```python
from build123d import *

# Parameters (mm, degrees)
BOSS_EXTRUDE1_DEPTH           = 1.8
EXTRUDE_THIN1_START           = 1.8
EXTRUDE_THIN1_DEPTH           = 3
SKETCH7_R                     = 1.55
SKETCH7_R_2                   = 0.01
EXTRUDE_THIN2_DEPTH           = 3.2
EXTRUDE_THIN2_DRAFT           = 5
EXTRUDE_THIN2_PROFILE_2_DEPTH = 3.2
EXTRUDE_THIN2_PROFILE_2_DRAFT = 5
EXTRUDE_THIN2_PROFILE_3_DEPTH = 3.2
EXTRUDE_THIN2_PROFILE_3_DRAFT = 5
EXTRUDE_THIN2_PROFILE_4_DEPTH = 3.2
EXTRUDE_THIN2_PROFILE_4_DRAFT = 5


with BuildPart() as part:
    # Sketch1 → Boss-Extrude1 (new body)
    with BuildSketch(Plane(origin=(0, 0, 0), x_dir=(0, 1, 0), z_dir=(0, 0, 1))):
        Polygon((40.609900374, 53.452613812), (-31.190099626, 53.452613812), (-31.190099626, -5.547386188), (40.609900374, -5.547386188), (40.609900374, -0.297386188), (43.209900374, 2.202613812), (43.109900374, 34.902613812), (40.609900374, 37.502613812), align=None)
    extrude(amount=BOSS_EXTRUDE1_DEPTH)

    # Sketch5 → Extrude-Thin1 (add)
    with BuildSketch(Plane(origin=(0, 0, 0), x_dir=(0, 1, 0), z_dir=(0, 0, 1)).offset(EXTRUDE_THIN1_START)):
        Polygon((-29.390099626, 51.652613812), (-29.390099626, -3.747386188), (38.809900374, -3.747386188), (38.809900374, -0.88342499), (41.360418353, 1.616884702), (41.360418353, 35.141633158), (38.809900374, 37.64194285), (38.809900374, 51.652613812), align=None)
        Polygon((-28.590099626, 50.852613812), (-28.590099626, -2.947386188), (38.009900374, -2.947386188), (38.009900374, -0.547386188), (40.560418353, 1.952923505), (40.560418353, 34.805594355), (38.009900374, 37.305904047), (38.009900374, 50.852613812), align=None, mode=Mode.SUBTRACT)
    extrude(amount=EXTRUDE_THIN1_DEPTH)


with BuildPart() as extrude_thin2_tool:
    # Sketch7 → Extrude-Thin2 (with draft: the straight prism first)
    with BuildSketch(Plane.XY.offset(1.8)):
        with Locations((-4.802613812, 37.960418353)):
            Circle(SKETCH7_R)
        with Locations((-4.802613812, 37.960418353)):
            Circle(SKETCH7_R_2, mode=Mode.SUBTRACT)
    extrude(amount=EXTRUDE_THIN2_DEPTH)
    # Extrude-Thin2: the draft: its side faces are tilted about the plane it starts from
    extrude_thin2_sides = [extrude_thin2_tool.faces().sort_by_distance(p)[0] for p in [
        (-6.352613812, 37.960418353, 3.4),
        (-4.812613812, 37.960418353, 3.4),
    ]]
    draft(extrude_thin2_sides, Plane.XY.offset(1.8), EXTRUDE_THIN2_DRAFT)


with BuildPart() as part_1:
    add(part.part)

    # Extrude-Thin2: add extrude_thin2_tool
    add(extrude_thin2_tool.part)


with BuildPart() as extrude_thin2_profile_2_tool:
    # Sketch7 → Extrude-Thin2 profile 2 (with draft: the straight prism first)
    with BuildSketch(Plane.XY.offset(1.8)):
        with Locations((-32.702613812, 37.960418353)):
            Circle(SKETCH7_R)
        with Locations((-32.702613812, 37.960418353)):
            Circle(SKETCH7_R_2, mode=Mode.SUBTRACT)
    extrude(amount=EXTRUDE_THIN2_PROFILE_2_DEPTH)
    # Extrude-Thin2 profile 2: the draft: its side faces are tilted about the plane it starts from
    extrude_thin2_profile_2_sides = [extrude_thin2_profile_2_tool.faces().sort_by_distance(p)[0] for p in [
        (-34.252613812, 37.960418353, 3.4),
        (-32.712613812, 37.960418353, 3.4),
    ]]
    draft(extrude_thin2_profile_2_sides, Plane.XY.offset(1.8), EXTRUDE_THIN2_PROFILE_2_DRAFT)


with BuildPart() as part_2:
    add(part_1.part)

    # Extrude-Thin2 profile 2: add extrude_thin2_profile_2_tool
    add(extrude_thin2_profile_2_tool.part)


with BuildPart() as extrude_thin2_profile_3_tool:
    # Sketch7 → Extrude-Thin2 profile 3 (with draft: the straight prism first)
    with BuildSketch(Plane.XY.offset(1.8)):
        with Locations((0.297386188, -14.140099626)):
            Circle(SKETCH7_R)
        with Locations((0.297386188, -14.140099626)):
            Circle(SKETCH7_R_2, mode=Mode.SUBTRACT)
    extrude(amount=EXTRUDE_THIN2_PROFILE_3_DEPTH)
    # Extrude-Thin2 profile 3: the draft: its side faces are tilted about the plane it starts from
    extrude_thin2_profile_3_sides = [extrude_thin2_profile_3_tool.faces().sort_by_distance(p)[0] for p in [
        (-1.252613812, -14.140099626, 3.4),
        (0.287386188, -14.140099626, 3.4),
    ]]
    draft(extrude_thin2_profile_3_sides, Plane.XY.offset(1.8), EXTRUDE_THIN2_PROFILE_3_DRAFT)


with BuildPart() as part_3:
    add(part_2.part)

    # Extrude-Thin2 profile 3: add extrude_thin2_profile_3_tool
    add(extrude_thin2_profile_3_tool.part)


with BuildPart() as extrude_thin2_profile_4_tool:
    # Sketch7 → Extrude-Thin2 profile 4 (with draft: the straight prism first)
    with BuildSketch(Plane.XY.offset(1.8)):
        with Locations((-48.102613812, -13.040099626)):
            Circle(SKETCH7_R)
        with Locations((-48.102613812, -13.040099626)):
            Circle(SKETCH7_R_2, mode=Mode.SUBTRACT)
    extrude(amount=EXTRUDE_THIN2_PROFILE_4_DEPTH)
    # Extrude-Thin2 profile 4: the draft: its side faces are tilted about the plane it starts from
    extrude_thin2_profile_4_sides = [extrude_thin2_profile_4_tool.faces().sort_by_distance(p)[0] for p in [
        (-49.652613812, -13.040099626, 3.4),
        (-48.112613812, -13.040099626, 3.4),
    ]]
    draft(extrude_thin2_profile_4_sides, Plane.XY.offset(1.8), EXTRUDE_THIN2_PROFILE_4_DRAFT)


with BuildPart() as part_4:
    add(part_3.part)

    # Extrude-Thin2 profile 4: add extrude_thin2_profile_4_tool
    add(extrude_thin2_profile_4_tool.part)


solid = part_4.part
```
Read the model definition and answer for the solid it produces. Units are mm, in the model's axes. A direction names the side the tool comes from. Coordinates: 2 decimals unless noted, no trailing zeros. Order: outer loops, then holes, each group sorted by start corner. A loop starts at its lowest first (then second) coordinate and runs counter-clockwise, first axis right, second up. Notation, with made-up numbers: (-34.75, -19) - (-27.75, -19) arc R38 cw to (-27.75, 20) - close; hole circle Ø4 at (2, 68.5). An arc over 180 degrees is marked (long way). Answer as a JSON object with one key per item and string values. Group by question number.
Item 1: Consider probe 1 along Y at (x, z) = (-38, 2.2); probe 2 along Y at (x, z) = (-18, 3.25); probe 3 along X at (y, z) = (19.5, 3.75). Determine where each line is inside the solid, lowest interval first. Write a range as from..to.
Item 2: The mould has two halves that part along Y. Classify faces 4 (the face through (-44, 38.01, 3)), 5 (the face through (-32, 38, 5)), 6 (the face through (-45, 40.61, 1)): +Y half, -Y half, draft (parallel to the pull), parting line (faces both ways), or undercut.
Item 3: A tool of negligible diameter and unlimited length cuts with its end or side. For faces 1 (the face through (-45, 38.81, 3)), 2 (the face through (3, 40.61, 1)), 3 (the face through (-36.04, 39.3, 3.28)), from which of +Z, -Z, +X, -X, +Y, -Y can it reach the whole face along a straight path? Write none if from no direction.
Item 4: Section C-C (y = 22.5) is taken. Give the vertices of the cut face in (x, z).
Item 5: Section A-A (z = 3.3) is taken. State how many separate pieces and enclosed holes the cut face has, plus the area to 3 significant figures.
Item 6: Flat-ended cylindrical pins translate along their axes: P1, Ø0.9, axis at y = -9.5, z = 2.5, coming from the -X side; P2, Ø1.5, axis at y = 0, z = 3, coming from the +X side; P3, Ø1, axis at x = -5.5, z = 3.5, coming from the +Y side. Find the tip coordinate at first contact, or state that the pin passes through.
Item 7: Section B-B (x = -44) is taken. Give the vertices of the cut face in (y, z), plus the area to 3 significant figures.
Results are:
{
 "1": {"probe 1": "y = -29.39..-28.59, 38.01..38.81", "probe 2": "y = -29.39..-28.59, 40.56..41.36", "probe 3": "x = -51.65..-50.85, 2.95..3.75"},
 "2": {"face 4": "undercut", "face 5": "draft", "face 6": "+Y half"},
 "3": {"face 1": "+Z, -X, +Y", "face 2": "+Z, -Z, +X, +Y", "face 3": "+Z"},
 "4": {"outline": "(-53.45, 0) - (5.55, 0) - (5.55, 1.8) - (3.75, 1.8) - (3.75, 4.8) - (2.95, 4.8) - (2.95, 1.8) - (-50.85, 1.8) - (-50.85, 4.8) - (-51.65, 4.8) - (-51.65, 1.8) - (-53.45, 1.8) - close"},
 "5": {"separate pieces": "5", "enclosed holes": "5", "area": "222 mm^2"},
 "6": {"P1": "stops at x = -51.65", "P2": "stops at x = 3.75", "P3": "stops at y = 41.36"},
 "7": {"outline": "(-31.19, 0) - (40.61, 0) - (40.61, 1.8) - (38.81, 1.8) - (38.81, 4.8) - (38.01, 4.8) - (38.01, 1.8) - (-28.59, 1.8) - (-28.59, 4.8) - (-29.39, 4.8) - (-29.39, 1.8) - (-31.19, 1.8) - close", "area": "134 mm^2"}
}
